Could you check a few things on this model? Use its own coordinates, in mm. Face numbers are marked on the shaded views. A direction names the side the tool comes from. Round coordinates to 2 decimals unless told otherwise and drop trailing zeros. Write each loop counter-clockwise with the first axis right and the second up, starting at its lowest first coordinate (ties: lowest second). Pieces come first, ordered by that corner, then holes. Notation, with made-up numbers: (12.25, 18.25) -> (27.25, 18.25) arc R25 cw to (27.25, 55.25) -> close; hole circle Ø7 at (3, 67). An arc over 180 degrees is marked (long way). One line per question, with ' | ' between items. Start each with the question number.
1. If I drill on line 1 along X through (y, z) = (1.6, 6.5); line 2 along Z through (x, y) = (-2.25, -0.6); line 3 along Y through (x, z) = (-1.95, -8.5), over which ranges is the centre line in solid material (lowest first)? Write a range as [from, to].
2. Imagine slicing it at A-A, the plane y = 0. List the corners of the cut face in (x, z) for me.
3. For pin 1 Ø1 at (x, z) = (-1, -27) entering from -Y; pin 2 Ø1.1 at (y, z) = (0.5, 4) entering from +X; pin 3 Ø3 at (x, y) = (2, 1) entering from -Z; pin 4 Ø1.9 at (y, z) = (0.5, 2.5) entering from -X, each with a flat end and sliding along its axis, tell me the tip position at first contact or that it passes through.
4. Imagine slicing it at B-B, the plane x = -1. List the corners of the cut face in (y, z) for me, and give its area (3 significant figures).
5. Imagine slicing it at C-C, the plane z = -12.5. List the corners of the cut face in (x, y) for me.
6. For the marked faces 1, 2 and 3, which set-ups out of +Z, -Z, +X, -X, +Y, -Y let a thin tool reach every point of the face, with its end or its side?
from build123d import *

# Parameters (mm, degrees)
SKETCH_1_W      = 2.6
SKETCH_1_H      = 14.5
EXTRUDE_1_DEPTH = 7.8


with BuildPart() as part:
    # 草图1 → 旋转1 (revolve)
    with BuildSketch(Plane(origin=(0, 0, 0), x_dir=(1, 0, 0), z_dir=(0, 1, 0))):
        with Locations((1.3, 7.25)):
            Rectangle(SKETCH_1_W, SKETCH_1_H)
    revolve(axis=Axis((0, 0, 0), (0, 0, -1)))

    # 草图2 → 凸台-拉伸1 (add)
    with BuildSketch(Plane.XY):
        with BuildLine():
            Line((-1.75, 1.9), (-1.75, -1.9))
            ThreePointArc((-1.75, -1.9), (0, -2.5), (1.75, -1.9))
            Line((1.75, -1.9), (1.75, 1.9))
            ThreePointArc((1.75, 1.9), (0, 2.5), (-1.75, 1.9))
        make_face()
    extrude(amount=EXTRUDE_1_DEPTH)

    # 镜向1: part across plane


with BuildPart() as part_1:
    add(part.part)
    add(part.part.mirror(Plane(origin=(0, 0, -14.5), x_dir=(1, 0, 0), z_dir=(0, 0, -1))))


solid = part_1.part
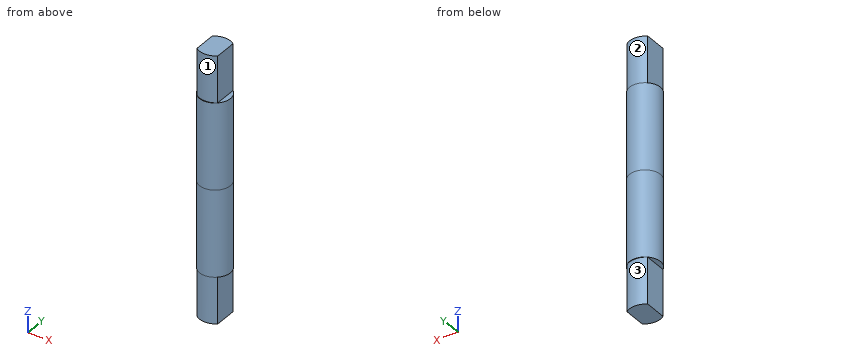
Geometry results:
1) line 1: x = [-1.75, 1.75] | line 2: z = [-29, 0] | line 3: y = [-1.72, 1.72]
2) outline: (-2.6, -29) -> (-1.75, -29) -> (-1.75, -36.8) -> (1.75, -36.8) -> (1.75, -29) -> (2.6, -29) -> (2.6, 0) -> (1.75, 0) -> (1.75, 7.8) -> (-1.75, 7.8) -> (-1.75, 0) -> (-2.6, 0) -> close
3) pin 1: stops at y = -2.55 | pin 2: stops at x = 1.75 | pin 3: stops at z = -36.8 | pin 4: stops at x = -1.75
4) outline: (-2.4, -29) -> (-2.32, -29) -> (-2.32, -36.8) -> (2.32, -36.8) -> (2.32, -29) -> (2.4, -29) -> (2.4, 0) -> (2.32, 0) -> (2.32, 7.8) -> (-2.32, 7.8) -> (-2.32, 0) -> (-2.4, 0) -> close | area: 212 mm2
5) outline: circle Ø5.2 at (0, 0)
6) face 1: +Z, -Y | face 2: +Z, +Y | face 3: -Z, +Y
